Part print with two shaded views. Sizes in mm from the minimum x, y, z corner. Give positions to 0.01 mm unless a question says otherwise; leave off trailing zeros. Order: outer loops, then holes, each group sorted by start corner. A loop starts at its lowest first (then second) coordinate and runs counter-clockwise, first axis right, second up. Notation, with made-up numbers: M 68,-9 L 112,-9 A31 ccw 112,27 Z; hole C 39,-24 d3. An arc over 180 degrees is marked long. Return JSON: item names as keys, results as strings.
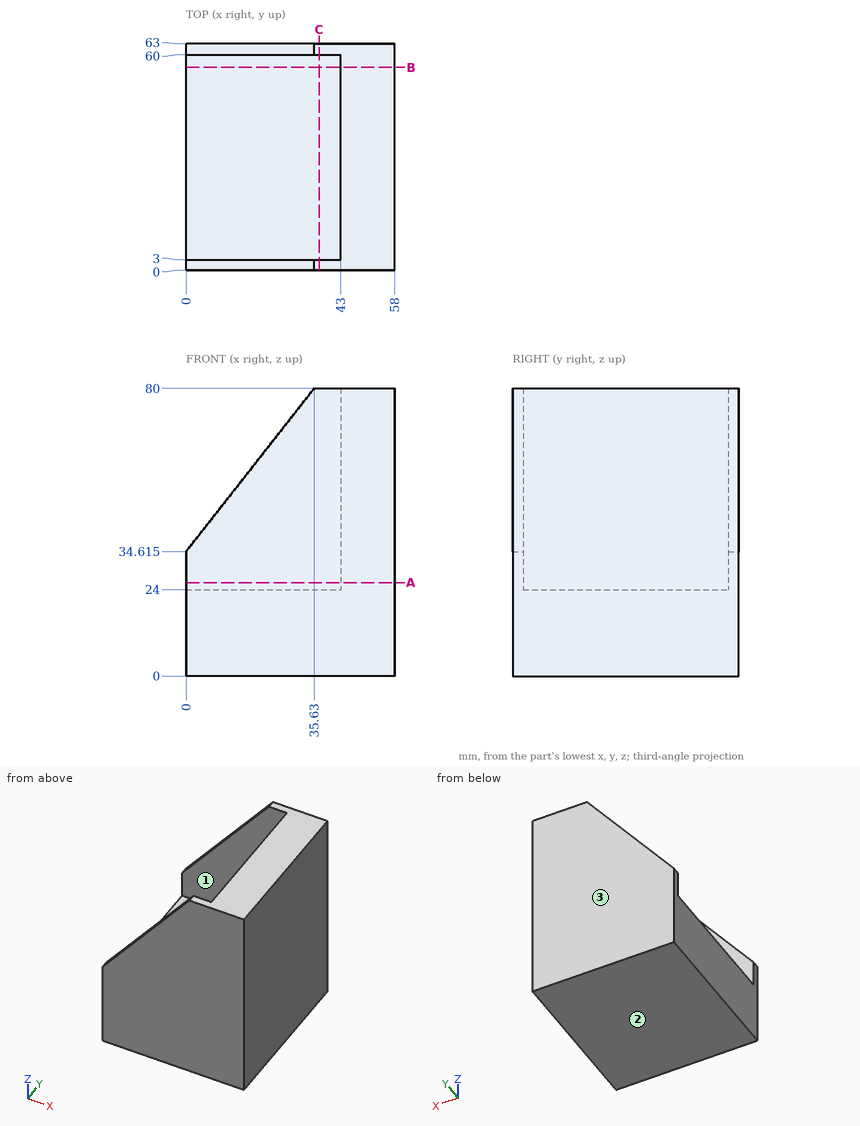
Q1. Probe line 1 along Y through (x, z) = (24, 41); line 2 along X through (y, z) = (17, 31.5); line 3 along Z through (x, y) = (40, 32). List the from-to ranges inside material, lowest first.
Established:
{"line 1": "y = 0 to 3, 60 to 63", "line 2": "x = 43 to 58", "line 3": "z = 0 to 24"}
Q2. Band-saw the part on A-A (z = 26). Give the cut face in (x, y), then the cut area to 3 significant figures.
Established:
{"outline": "M 0,0 L 58,0 L 58,63 L 0,63 L 0,60 L 43,60 L 43,3 L 0,3 Z", "area": "1,200 mm²"}
Q3. Band-saw the part on B-B (y = 56.5). Give the cut face in (x, z).
Established:
{"outline": "M 0,0 L 58,0 L 58,80 L 43,80 L 43,24 L 0,24 Z"}
Q4. Band-saw the part on C-C (x = 37). Give the cut face in (y, z), then the cut area to 3 significant figures.
Established:
{"outline": "M 0,0 L 63,0 L 63,80 L 60,80 L 60,24 L 3,24 L 3,80 L 0,80 Z", "area": "1,850 mm²"}
Q5. Two-plate mould, pull along Y, no slides. Class the marked faces 1, 2 and 3: +Y half, -Y half, draft (parallel to the pull), parting line (faces both ways), or undercut.
Established:
{"face 1": "undercut", "face 2": "draft", "face 3": "+Y half"}
Q6. Pin check, flat tips, straight feed: pin 1 (6 mm diameter, centred on x = 44.5, y = 39.5, fed in from -Z); pin 2 (4 mm diameter, centred on y = 49, z = 44, fed in from -X). Stop position of each tip, or through.
Established:
{"pin 1": "stops at z = 0", "pin 2": "stops at x = 43"}
